Read the model definition and answer for the solid it produces. Units are mm, in the model's axes. Coordinates: 2 decimals unless noted, no trailing zeros. Order: outer loops, then holes, each group sorted by start corner. A loop starts at its lowest first (then second) coordinate and runs counter-clockwise, first axis right, second up.
from build123d import *

# Parameters (mm, degrees)
SKETCH1_R           = 4
SKETCH1_R_2         = 10
BOSS_EXTRUDE1_DEPTH = 3
FILLET1_R           = 30


with BuildPart() as part:
    # Sketch1 → Boss-Extrude1 (new body)
    with BuildSketch(Plane.XY):
        with BuildLine():
            Line((-11.149584488, -35), (-11.149584488, -11.149584488))
            Line((-11.149584488, -11.149584488), (-35, -11.149584488))
            ThreePointArc((-35, -11.149584488), (-46.149584488, 0), (-35, 11.149584488))
            Line((-35, 11.149584488), (-11.149584488, 11.149584488))
            Line((-11.149584488, 11.149584488), (-11.149584488, 35))
            ThreePointArc((-11.149584488, 35), (0, 46.149584488), (11.149584488, 35))
            Line((11.149584488, 35), (11.149584488, 11.149584488))
            Line((11.149584488, 11.149584488), (35, 11.149584488))
            ThreePointArc((35, 11.149584488), (46.149584488, 0), (35, -11.149584488))
            Line((35, -11.149584488), (11.149584488, -11.149584488))
            Line((11.149584488, -11.149584488), (11.149584488, -35))
            ThreePointArc((11.149584488, -35), (0, -46.149584488), (-11.149584488, -35))
        make_face()
        with Locations((-35, 0)):
            Circle(SKETCH1_R, mode=Mode.SUBTRACT)
        with Locations((35, 0)):
            Circle(SKETCH1_R, mode=Mode.SUBTRACT)
        with Locations((0, 35)):
            Circle(SKETCH1_R, mode=Mode.SUBTRACT)
        with Locations((0, -35)):
            Circle(SKETCH1_R, mode=Mode.SUBTRACT)
        Circle(SKETCH1_R_2, mode=Mode.SUBTRACT)
    extrude(amount=BOSS_EXTRUDE1_DEPTH)

    # Fillet1
    fillet1_edges = [part.edges().sort_by_distance(p)[0] for p in [
        (-11.149584488, 11.149584488, 1.5),
        (11.149584488, 11.149584488, 1.5),
        (11.149584488, -11.149584488, 1.5),
        (-11.149584488, -11.149584488, 1.5),
    ]]
    fillet(fillet1_edges, radius=FILLET1_R)


solid = part.part
Q1. Straight lines are drawn through the part: L1, parallel to X at y = -9, z = 0.55; L2, parallel to Y at x = 35, z = 1.05; L3, parallel to Y at x = 8.5, z = 0.8. For each, find the intervals that lie inside material, in ascending order.
Q2. Determine the mould class of faces 1 (the cylindrical face through (-0.521, -31.034, 1.479)), 2 (the cylindrical face through (0.223, -46.147, 1.479)), 3 (the flat face through (-10, -10, 0)) for opening direction Y: +Y half, -Y half, draft (parallel to the pull), parting line (faces both ways), or undercut.
Q3. The part is cut by section C-C, the plane z = 0.9. State how many separate pieces and enclosed holes the cut face has, then the cut area to 3 significant figures.
Q4. The part is cut by section A-A, the plane x = 0. Determine the outline of the cut face in (y, z).
Q5. This flat-tipped pin is pushed along its axis until it touches: P1, Ø1, axis at x = 4.5, z = 1, coming from the +Y side. Where does it stop, or does it pass through?
Computed values:
1. L1: x = -41.58 to -4.36, 4.36 to 41.58
1. L2: y = -11.3 to -4, 4 to 11.3
1. L3: y = -42.22 to -5.27, 5.27 to 42.22
2. face 1: undercut
2. face 2: -Y half
2. face 3: draft
3. separate pieces: 1
3. enclosed holes: 5
3. area: 3,580 mm2
4. outline: (-46.15, 0) - (-39, 0) - (-39, 3) - (-46.15, 3) - close; (-31, 0) - (-10, 0) - (-10, 3) - (-31, 3) - close; (10, 0) - (31, 0) - (31, 3) - (10, 3) - close; (39, 0) - (46.15, 0) - (46.15, 3) - (39, 3) - close
5. P1: stops at y = 45.41
